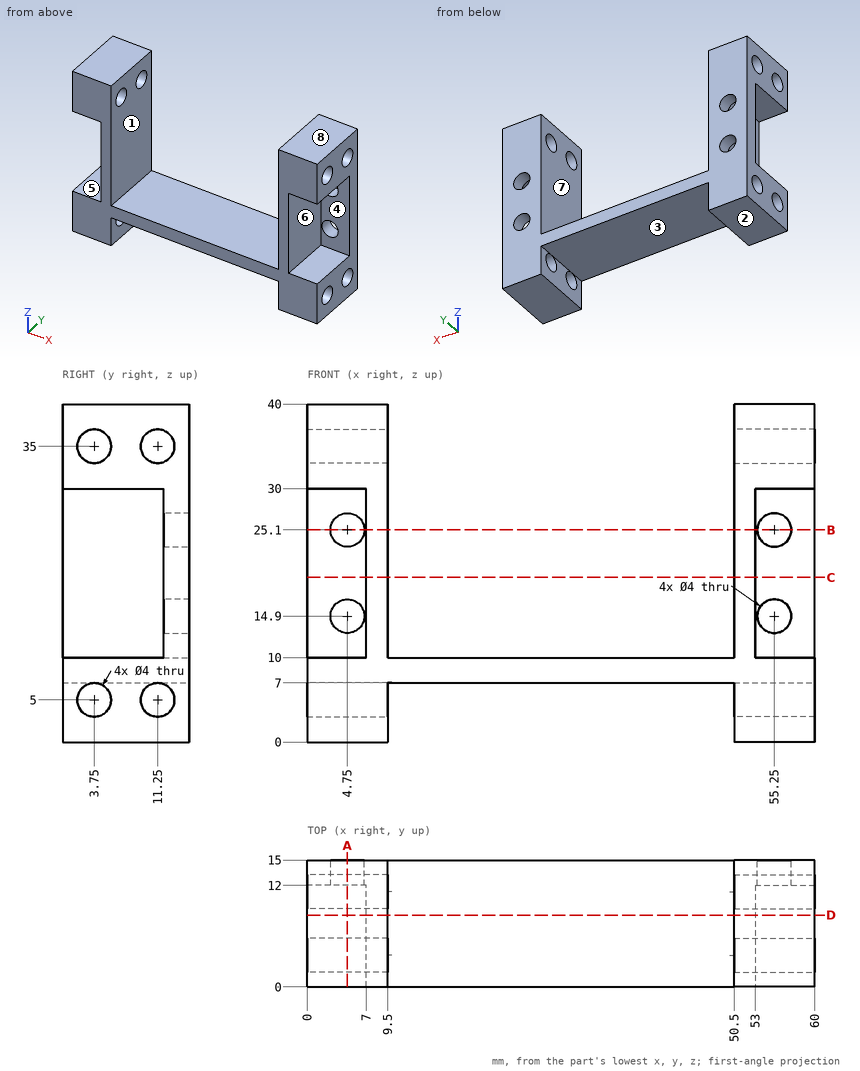
Input: dimensioned drawing with shaded views. Units: mm. Origin: part minimum x, y, z. A direction names the side the tool comes from. Round coordinates to 2 decimals unless told otherwise and drop trailing zeros. Order: outer loops, then holes, each group sorted by start corner. A loop starts at its lowest first (then second) coordinate and runs counter-clockwise, first axis right, second up. Notation, with made-up numbers: (56, 12.25) - (73, 12.25) arc R23 cw to (73, 22.25) - close; hole circle Ø3 at (30.5, 71.5). An arc over 180 degrees is marked (long way). Use CSV: the item, a comma, the result in double quotes. Start each with the question number.
Q1. Section query A-A (x = 4.75). Return loops of the section in (y, z).
Q2. Access query for the marked faces 1, 2, 3, 4 and 5. Directions: +Z, -Z, +X, -X, +Y, -Y. A direction counts if a zero-diameter tool reaches every point of the face in a straight line with its end or side. Return the directions, or none.
Q3. Section query B-B (z = 25.1). Return loops of the section in (x, y), and give its area (3 significant figures).
Q4. Section query D-D (y = 8.5). Return loops of the section in (x, z).
Q5. Mould query, pull axis X, two halves, no side actions, for the marked faces 6, 7 and 8. Classes: +X half, -X half, draft (parallel to the pull), parting line (faces both ways), or undercut.
Q6. Section query C-C (z = 19.5). Return loops of the section in (x, y).
Q7. First-contact query: pin 1 (4.5 mm diameter, centred on x = 34, y = 9.5, fed in from -Z); pin 2 (4 mm diameter, centred on y = 5.5, z = 25, fed in from -X); pin 3 (4.5 mm diameter, centred on x = 26.5, y = 6, fed in from +Z). Flat tips, straight axial feed; report the tip coordinate or a pass-through.
Q8. Material intervals for line 1 along Z through (x, y) = (55.25, 13.7); line 2 along Y through (x, z) = (57, 5); line 3 along Z through (x, y) = (54.25, 3.75), sorted ascending. Write a range as from..to.
Result set:
1,outline,"(0, 0) - (15, 0) - (15, 12.9) - (12, 12.9) - (12, 10) - (0, 10) - close; (0, 30) - (12, 30) - (12, 27.1) - (15, 27.1) - (15, 40) - (0, 40) - close; (12, 16.9) - (15, 16.9) - (15, 23.1) - (12, 23.1) - close; hole circle Ø4 at (3.75, 5); hole circle Ø4 at (3.75, 35); hole circle Ø4 at (11.25, 5); hole circle Ø4 at (11.25, 35)"
2,face 1,"+Z, +Y, -Y"
2,face 2,"-Z, +X, -X, +Y, -Y"
2,face 3,"-Z, +Y, -Y"
2,face 4,"+X, -Y"
2,face 5,"-X, -Y"
3,outline,"(0, 12) - (2.75, 12) - (2.75, 15) - (0, 15) - close; (6.75, 12) - (7, 12) - (7, 0) - (9.5, 0) - (9.5, 15) - (6.75, 15) - close; (50.5, 0) - (53, 0) - (53, 12) - (53.25, 12) - (53.25, 15) - (50.5, 15) - close; (57.25, 12) - (60, 12) - (60, 15) - (57.25, 15) - close"
3,area,"93.0 mm2"
4,outline,"(0, 0) - (9.5, 0) - (9.5, 7) - (50.5, 7) - (50.5, 0) - (60, 0) - (60, 10) - (53, 10) - (53, 30) - (60, 30) - (60, 40) - (50.5, 40) - (50.5, 10) - (9.5, 10) - (9.5, 40) - (0, 40) - (0, 30) - (7, 30) - (7, 10) - (0, 10) - close"
5,face 6,"+X half"
5,face 7,"undercut"
5,face 8,"draft"
6,outline,"(0, 12) - (7, 12) - (7, 0) - (9.5, 0) - (9.5, 15) - (0, 15) - close; (50.5, 0) - (53, 0) - (53, 12) - (60, 12) - (60, 15) - (50.5, 15) - close"
7,pin 1,"stops at z = 7"
7,pin 2,"stops at x = 7"
7,pin 3,"stops at z = 10"
8,line 1,"z = 0..12.9, 16.9..23.1, 27.1..40"
8,line 2,"y = 0..1.75, 5.75..9.25, 13.25..15"
8,line 3,"z = 0..3, 7..10, 30..33, 37..40"
